For this review, use the dimensioned drawing (mm, ordinates from the lowest corner) and the shaded views. A direction names the side the tool comes from. Give positions to 0.01 mm unless a question says otherwise; leave off trailing zeros. Order: outer loops, then holes, each group sorted by start corner. A loop starts at its lowest first (then second) coordinate and runs counter-clockwise, first axis right, second up. Notation, with made-up numbers: (8, 64.5) -> (55, 64.5) arc R12 cw to (55, 82.5) -> close; hole circle Ø7 at (-35.5, 35.5). An arc over 180 degrees is marked (long way). One line per item, written item: value. Start each with the question number.
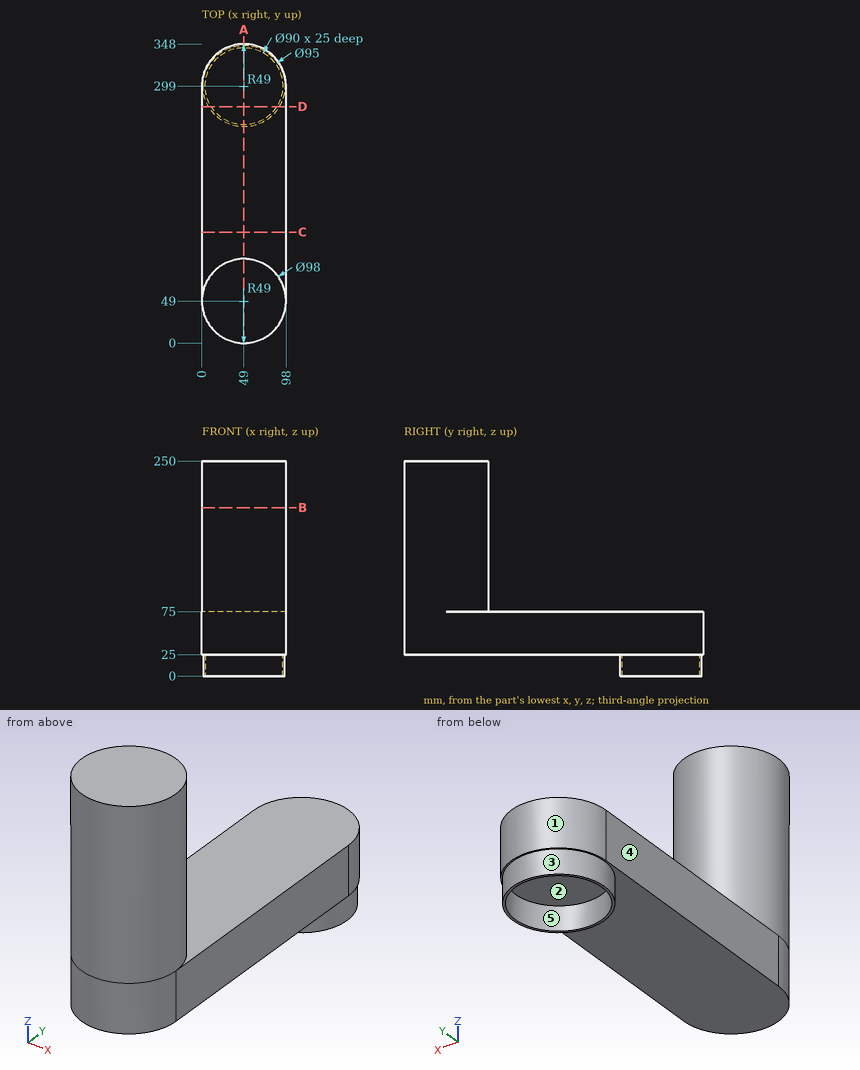
Q1. For the marked faces 1 and 2, list the 3-axis set-ups (+Z, -Z, +X, -X, +Y, -Y) from which the entire face can be reached by the end or side of a thin tool; tool diameter is ignored.
Q2. Take a section at A-A (x = 49). State the section outline as (y, z) points, and give its area (3 significant figures).
Q3. Mouldability with a two-part tool opening along Y and no side actions: class the marked faces 3, 4 and 5 as pulls with the +Y half, pulls with the -Y half, needs draft (parallel to the pull), parting line crosses it, or undercut.
Q4. Take a section at D-D (y = 275). State the section outline as (x, z) points.
Q5. Take a section at B-B (z = 196). State the section outline as (x, y) points.
Q6. For pin 1 Ø12 at (x, z) = (53, 110.5) entering from +Y; pin 2 Ø3 at (x, y) = (57.5, 128) entering from +Z; pin 3 Ø10 at (x, y) = (54, 153) entering from -Z, all flat-tipped, find the tip position at first contact; note any pin that passes through.
Q7. For line 1 along Y through (x, z) = (49, 19); line 2 along Z through (x, y) = (27.5, 86); line 3 along Z through (x, y) = (91, 180), list the stretches that pass through material, from the lowest coordinate up.
Q8. Take a section at C-C (y = 129). State the section outline as (x, z) points.
Answers below:
1. face 1: +Z, -Z, +Y
1. face 2: -Z
2. outline: (0, 25) -> (251.5, 25) -> (251.5, 0) -> (254, 0) -> (254, 25) -> (344, 25) -> (344, 0) -> (346.5, 0) -> (346.5, 25) -> (348, 25) -> (348, 75) -> (98, 75) -> (98, 250) -> (0, 250) -> close
2. area: 34,700 mm²
3. face 3: parting line crosses it
3. face 4: needs draft
3. face 5: undercut
4. outline: (0, 25) -> (8.01, 25) -> (8.01, 0) -> (10.93, 0) -> (10.93, 25) -> (87.07, 25) -> (87.07, 0) -> (89.99, 0) -> (89.99, 25) -> (98, 25) -> (98, 75) -> (0, 75) -> close
5. outline: circle Ø98 at (49, 49)
6. pin 1: stops at y = 98
6. pin 2: stops at z = 75
6. pin 3: stops at z = 25
7. line 1: y = 251.5 to 254, 344 to 346.5
7. line 2: z = 25 to 250
7. line 3: z = 25 to 75
8. outline: (0, 25) -> (98, 25) -> (98, 75) -> (0, 75) -> close
